Geometry: final body of the model. Coordinates: model frame, mm. Face numbers are marked on the shaded views. A direction names the side the tool comes from. Coordinates: 2 decimals unless noted, no trailing zeros. Order: outer loops, then holes, each group sorted by start corner. A loop starts at its lowest first (then second) coordinate and runs counter-clockwise, first axis right, second up. Notation, with made-up numbers: M -17.75,48 L 9.25,48 A23 ccw 9.25,66 Z; hole C 20,53.25 d6. An arc over 180 degrees is marked long. Use CSV: the item, a comma, the result in double quotes. Start each with the question number.
Q1. Access query for the marked faces 1 and 2. Directions: +Z, -Z, +X, -X, +Y, -Y. A direction counts if a zero-diameter tool reaches every point of the face in a straight line with its end or side. Return the directions, or none.
Q2. Section query A-A, the plane y = 0. Output: boundary loops of the cut face in (x, z), and give its area (3 significant figures).
Q3. Ray query, probe 1 along Y at (x, z) = (0, 94); probe 2 along Y at (x, z) = (-3.75, 189); probe 3 along X at (y, z) = (-2.75, 67). Return the intervals inside material, ascending.
Q4. Section query C-C, the plane z = 139. Output: boundary loops of the cut face in (x, y).
Q5. First-contact query: P1, Ø2, axis at y = 2, z = 111.5, coming from the -X side; P2, Ø2, axis at x = 0.5, z = 53.5, coming from the +Y side; P3, Ø5, axis at y = -3, z = 131, coming from the +X side; P4, Ø11, axis at x = 2.5, y = -2, coming from the -Z side. Flat tips, straight axial feed; report the tip coordinate or a pass-through.
Q6. Section query B-B, the plane x = 0. Output: boundary loops of the cut face in (y, z), and give its area (3 significant figures).
from build123d import *

# Parameters (mm, degrees)
SKETCH2_R           = 8
SKETCH2_R_2         = 7
BOSS_EXTRUDE1_DEPTH = 196
SKETCH3_R           = 8
BOSS_EXTRUDE2_DEPTH = 4
SKETCH6_R           = 10
BOSS_EXTRUDE3_DEPTH = 11.25


with BuildPart() as part:
    # Sketch2 → Boss-Extrude1 (new body)
    with BuildSketch(Plane.XY):
        Circle(SKETCH2_R)
        Circle(SKETCH2_R_2, mode=Mode.SUBTRACT)
    extrude(amount=BOSS_EXTRUDE1_DEPTH)

    # Sketch3 → Boss-Extrude2 (add)
    with BuildSketch(Plane.XY.offset(196)):
        Circle(SKETCH3_R)
    extrude(amount=BOSS_EXTRUDE2_DEPTH)

    # Sketch6 → Boss-Extrude3 (add, symmetric)
    with BuildSketch(Plane(origin=(0, 0, 0), x_dir=(1, 0, 0), z_dir=(0, 1, 0))):
        with Locations(Location((0, -206, 0), (0, 0, 270))):
            Circle(SKETCH6_R)
    extrude(amount=BOSS_EXTRUDE3_DEPTH, both=True)


solid = part.part
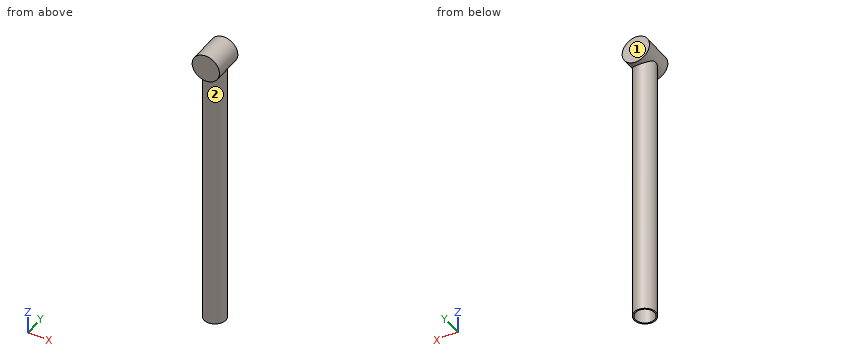
Responses:
1,face 1,"+Z, -Z, +X, -X, +Y"
1,face 2,"-Z"
2,outline,"M -8,0 L -7,0 L -7,196 L 7,196 L 7,0 L 8,0 L 8,200 A10 ccw long -8,200 Z"
2,area,"725 mm²"
3,probe 1,"y = -8 to -7, 7 to 8"
3,probe 2,"y = -7.07 to -5.91, 5.91 to 7.07"
3,probe 3,"x = -7.51 to -6.44, 6.44 to 7.51"
4,outline,"C 0,0 d16; hole C 0,0 d14"
5,P1,"stops at x = -7.94"
5,P2,"stops at y = 8"
5,P3,"stops at x = 7.98"
5,P4,"stops at z = 0"
6,outline,"M -11.25,196 L -8,196 L -8,0 L -7,0 L -7,196 L 7,196 L 7,0 L 8,0 L 8,196 L 11.25,196 L 11.25,216 L -11.25,216 Z"
6,area,"842 mm²"
